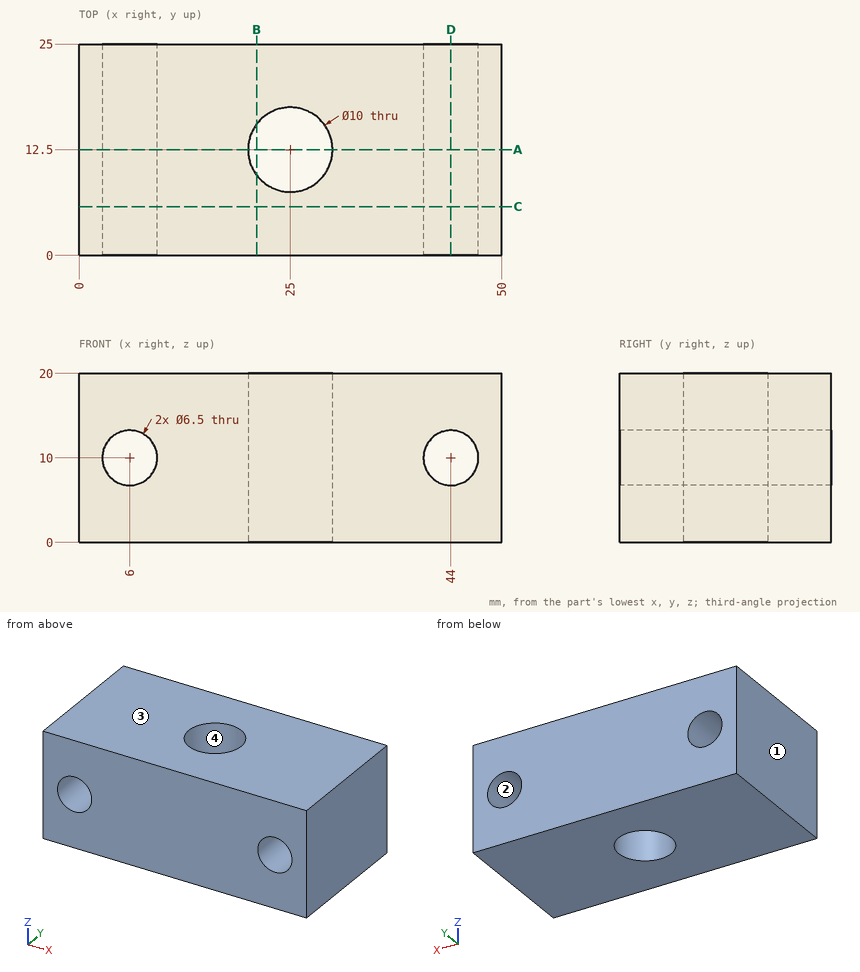
Study the drawing (mm; zero at the part's minimum x, y, z) and answer. Give positions to 0.01 mm unless a question says otherwise; leave off trailing zeros. Write each loop counter-clockwise with the first axis right and the second up, starting at its lowest first coordinate (ties: lowest second). Pieces come first, ordered by that corner, then holes. Notation, with made-up numbers: (59, 83) - (113, 83) arc R19 cw to (113, 98) - close; hole circle Ø6 at (-20.75, -36). An arc over 180 degrees is marked (long way). Write item = value, one per line. Start each with the question number.
Item 1: Find the intervals of material crossed by probe 1 along X at (y, z) = (17.75, 10.25); probe 2 along Y at (x, z) = (25, 7.25); probe 3 along Z at (x, y) = (6, 17.25), in increasing order. Write a range as [from, to].
Item 2: The mould has two halves that part along X. Classify the marked faces 1, 2, 3 and 4: +X half, -X half, draft (parallel to the pull), parting line (faces both ways), or undercut.
Item 3: Find section B-B (x = 21). Give the vertices of the cut face in (y, z).
Item 4: This flat-tipped pin is pushed along its axis until it touches: P1, Ø7.5, axis at x = 6, z = 10, coming from the +Y side. Where does it stop, or does it pass through?
Item 5: Find section D-D (x = 44). Give the vertices of the cut face in (y, z).
Item 6: Find section C-C (y = 5.75). Give the vertices of the cut face in (x, z), then the cut area to 3 significant figures.
Item 7: Find section A-A (y = 12.5). Give the vertices of the cut face in (x, z).
Response:
q1.probe_1 = [0, 2.76], [9.24, 40.76], [47.24, 50]
q1.probe_2 = [0, 7.5], [17.5, 25]
q1.probe_3 = [0, 6.75], [13.25, 20]
q2.face_1 = -X half
q2.face_2 = undercut
q2.face_3 = draft
q2.face_4 = undercut
q3.outline = (0, 0) - (9.5, 0) - (9.5, 20) - (0, 20) - close; (15.5, 0) - (25, 0) - (25, 20) - (15.5, 20) - close
q4.P1 = 25
q5.outline = (0, 0) - (25, 0) - (25, 6.75) - (0, 6.75) - close; (0, 13.25) - (25, 13.25) - (25, 20) - (0, 20) - close
q6.outline = (0, 0) - (50, 0) - (50, 20) - (0, 20) - close; hole circle Ø6.5 at (6, 10); hole circle Ø6.5 at (44, 10)
q6.area = 934 mm²
q7.outline = (0, 0) - (20, 0) - (20, 20) - (0, 20) - close; (30, 0) - (50, 0) - (50, 20) - (30, 20) - close; hole circle Ø6.5 at (6, 10); hole circle Ø6.5 at (44, 10)
